Input: part model. Units: mm. Frame: model coordinates. A direction names the side the tool comes from. Give positions to 0.01 mm unless a question says otherwise; leave off trailing zeros. Order: outer loops, then holes, each group sorted by start corner. A loop starts at its lowest first (then second) coordinate and runs counter-clockwise, first axis right, second up.
```python
from build123d import *

# Parameters (mm, degrees)
SKETCH_1_W                       = 167
SKETCH_1_H                       = 155
EXTRUDE_1_DEPTH                  = 4
FILLET_1_R                       = 9
FILLET_2_R                       = 18
CUT_EXTRUDE_1_REACH              = 115.993
HOLE_WIZARD_1_D                  = 5
HOLE_WIZARD_1_CBORE_D            = 8
HOLE_WIZARD_1_CBORE_DEPTH        = 1
EXTRUDE_3_DEPTH                  = 15
CUT_EXTRUDE_2_REACH              = 146.177
SKETCH_13_W                      = 6.5
SKETCH_13_H                      = 23
SKETCH_15_W                      = 8
SKETCH_15_H                      = 3
CUT_EXTRUDE_3_DEPTH              = 2.5
FILLET_3_R                       = 0.5
PATTERN_CIRCULAR_1_COUNT         = 4
FILLET_3_OF_PATTERN_CIRCULAR_1_R = 0.5
SKETCH_18_W                      = 10
SKETCH_18_H                      = 20
EXTRUDE_4_DEPTH                  = 2
FILLET_4_R                       = 1
FILLET_4_OF_MIRROR_1_R           = 1


with BuildPart() as part:
    # ｽｹｯﾁ1 → ﾎﾞｽ - 押し出し1 (new body)
    with BuildSketch(Plane.XY):
        Rectangle(SKETCH_1_W, SKETCH_1_H)
    extrude(amount=EXTRUDE_1_DEPTH)

    # ﾌｨﾚｯﾄ1
    fillet_1_edges = [part.edges().sort_by_distance(p)[0] for p in [
        (83.5, -77.5, 2),
        (83.5, 77.5, 2),
    ]]
    fillet(fillet_1_edges, radius=FILLET_1_R)

    # ﾌｨﾚｯﾄ2
    fillet_2_edges = [part.edges().sort_by_distance(p)[0] for p in [
        (-83.5, -77.5, 2),
        (-83.5, 77.5, 2),
    ]]
    fillet(fillet_2_edges, radius=FILLET_2_R)

    # ｽｹｯﾁ2 → ｶｯﾄ - 押し出し1 (cut, up to next)
    with BuildSketch(Plane.XY.offset(4), mode=Mode.PRIVATE) as cut_extrude_1_sk1:
        with BuildLine():
            Line((58.5, 77.5), (68.5, 77.5))
            Line((68.5, 77.5), (68.5, 72.5))
            ThreePointArc((68.5, 72.5), (63.5, 67.5), (58.5, 72.5))
            Line((58.5, 72.5), (58.5, 77.5))
        make_face()
    cut_extrude_1_tool1 = extrude(cut_extrude_1_sk1.sketch, amount=-CUT_EXTRUDE_1_REACH, mode=Mode.PRIVATE) & part.part
    add(cut_extrude_1_tool1.solids().sort_by_distance((63.5, 72.966749, 4))[0], mode=Mode.SUBTRACT)

    # 穴1 (through all)
    with Locations(Plane.XY.offset(4)):
        with Locations((66, 0)):
            CounterBoreHole(HOLE_WIZARD_1_D / 2, HOLE_WIZARD_1_CBORE_D / 2, HOLE_WIZARD_1_CBORE_DEPTH)

    # ｽｹｯﾁ11 → ﾎﾞｽ - 押し出し3 (add)
    with BuildSketch(Plane.XY.offset(4)):
        with BuildLine():
            Line((36.582099448, 12), (36.582099448, -12))
            ThreePointArc((36.582099448, -12), (-38.5, 0), (36.582099448, 12))
        make_face()
        with BuildLine():
            Line((34.641016151, 11.5), (34.641016151, -11.5))
            ThreePointArc((34.641016151, -11.5), (-36.5, 0), (34.641016151, 11.5))
        make_face(mode=Mode.SUBTRACT)
    extrude(amount=EXTRUDE_3_DEPTH)

    # ｽｹｯﾁ13 → ｶｯﾄ - 押し出し2 (cut, up to next)
    with BuildSketch(Plane(origin=(36.582099448, 0, 0), x_dir=(0, 0, -1), z_dir=(1, 0, 0)), mode=Mode.PRIVATE) as cut_extrude_2_sk1:
        with Locations((-13.75, 0)):
            Rectangle(SKETCH_13_W, SKETCH_13_H)
    cut_extrude_2_tool1 = extrude(cut_extrude_2_sk1.sketch, amount=-CUT_EXTRUDE_2_REACH, mode=Mode.PRIVATE) & part.part
    add(cut_extrude_2_tool1.solids().sort_by_distance((36.582099, 0, 13.75))[0], mode=Mode.SUBTRACT)

    # ｽｹｯﾁ15 → ｶｯﾄ - 押し出し3 (cut)
    with BuildSketch(Plane(origin=(-24.72592031, 24.748737342, 1.062480514), x_dir=(0.7076465964640425, 0.7064548659887622, 0.012562517011201728), z_dir=(-0.7064548659887622, 0.7071067811865462, 0.030356586119027387))):
        with Locations((0, -14.290598152)):
            Rectangle(SKETCH_15_W, SKETCH_15_H)
    cut_extrude_3 = extrude(amount=CUT_EXTRUDE_3_DEPTH, mode=Mode.SUBTRACT)

    # ﾌｨﾚｯﾄ3
    fillet_3_edges = [part.edges().sort_by_distance(p)[0] for p in [
        (-26.293687817, 26.037155642, 16.920446126),
        (-26.331375368, 26.1282254, 13.922065571),
    ]]
    fillet(fillet_3_edges, radius=FILLET_3_R)

    # 円形ﾊﾟﾀｰﾝ1: ｶｯﾄ - 押し出し3 ×4 about axis
    pattern_circular_1_axis = Axis((0, 0, 0), (0, 0, 1))
    for i in range(1, PATTERN_CIRCULAR_1_COUNT):
        add(cut_extrude_3.rotate(pattern_circular_1_axis, i * 360 / PATTERN_CIRCULAR_1_COUNT), mode=Mode.SUBTRACT)

    # ﾌｨﾚｯﾄ3 of 円形ﾊﾟﾀｰﾝ1
    fillet_3_of_pattern_circular_1_edges = [part.edges().sort_by_distance(p)[0] for p in [
        (-26.037155642, -26.293687817, 16.920446126),
        (-26.1282254, -26.331375368, 13.922065571),
        (26.293687817, -26.037155642, 16.920446126),
        (26.331375368, -26.1282254, 13.922065571),
        (26.037155642, 26.293687817, 16.920446126),
        (26.1282254, 26.331375368, 13.922065571),
    ]]
    fillet(fillet_3_of_pattern_circular_1_edges, radius=FILLET_3_OF_PATTERN_CIRCULAR_1_R)

    # ｽｹｯﾁ18 → ﾎﾞｽ - 押し出し4 (add)
    with BuildSketch(Plane(origin=(0, 0, 0), x_dir=(-1, 0, 0), z_dir=(0, 0, -1))):
        with Locations((-82.5, 45)):
            Rectangle(SKETCH_18_W, SKETCH_18_H)
    extrude_4 = extrude(amount=EXTRUDE_4_DEPTH)

    # ﾌｨﾚｯﾄ4
    fillet_4_edges = [part.edges().sort_by_distance(p)[0] for p in [
        (77.5, 45, -2),
    ]]
    fillet(fillet_4_edges, radius=FILLET_4_R)

    # ﾐﾗｰ1: ﾎﾞｽ - 押し出し4 across plane
    add(extrude_4.mirror(Plane.ZX))

    # ﾌｨﾚｯﾄ4 of ﾐﾗｰ1
    fillet_4_of_mirror_1_edges = [part.edges().sort_by_distance(p)[0] for p in [
        (77.5, -45, -2),
    ]]
    fillet(fillet_4_of_mirror_1_edges, radius=FILLET_4_OF_MIRROR_1_R)


solid = part.part
```
1) Pull-direction query (Y, two-part tool) for faces 1 (the face through (80.794, -74.934, 2.028)), 2 (the face through (64.85, -2.22, 1.48)), 3 (the face through (-26.18, 26.06, 14.06)), 4 (the face through (35, 0, 19)); classes: pulls with the +Y half, pulls with the -Y half, needs draft (parallel to the pull), parting line crosses it, or undercut.
2) Line query: probe 1 along Z at (x, y) = (-70.5, -25); probe 2 along Y at (x, z) = (0, 8.5); probe 3 along Y at (x, z) = (66, 3.75). Output: solid intervals per line, ascending.
3) Cut plane B-B (x = 66). Return the cut outline in (y, z).
4) Reachability of faces 5 (the face through (58.5, 75, 2)), 6 (the face through (26.06, 26.18, 14.06)), 7 (the face through (83.5, -1, 2)), 8 (the face through (64, -2, 3)) from +Z, -Z, +X, -X, +Y, -Y: full face, straight path, thin tool, end or side. Return the list, or none.
5) Cut plane A-A (y = 0). Return the cut outline in (x, z).
6) First-contact query: P1, Ø2, axis at x = 35.5, z = 14, coming from the -Y side; P2, Ø5, axis at x = 18, y = 34.5, coming from the -Z side; P3, Ø3, axis at x = 84.5, y = 49.5, coming from the +Z side; P4, Ø6, axis at x = -39.5, z = 5, coming from the -Y side. Flat tips, straight axial feed; report the tip coordinate or a pass-through.
7) Cut plane D-D (y = 49). Return the cut outline in (x, z).
8) Cut plane C-C (x = 0). Return the cut outline in (y, z).
Geometry says:
1. face 1: pulls with the -Y half
1. face 2: undercut
1. face 3: undercut
1. face 4: needs draft
2. probe 1: z = 0 to 4
2. probe 2: y = -38.5 to -36.5, 36.5 to 38.5
2. probe 3: y = -77.5 to -4, 4 to 68.17
3. outline: (-77.5, 0) - (-2.5, 0) - (-2.5, 3) - (-4, 3) - (-4, 4) - (-77.5, 4) - close; (2.5, 0) - (68.17, 0) - (68.17, 4) - (4, 4) - (4, 3) - (2.5, 3) - close
4. face 5: +Z, -Z, +Y
4. face 6: none
4. face 7: +Z, +X, +Y, -Y
4. face 8: +Z
5. outline: (-83.5, 0) - (63.5, 0) - (63.5, 3) - (62, 3) - (62, 4) - (36.58, 4) - (36.58, 10.5) - (34.64, 10.5) - (34.64, 4) - (-36.5, 4) - (-36.5, 19) - (-38.5, 19) - (-38.5, 4) - (-83.5, 4) - close; (34.64, 17) - (36.58, 17) - (36.58, 19) - (34.64, 19) - close; (68.5, 0) - (83.5, 0) - (83.5, 4) - (70, 4) - (70, 3) - (68.5, 3) - close
6. P1: stops at y = -17.09
6. P2: stops at z = 0
6. P3: stops at z = 4
6. P4: stops at y = -77.5
7. outline: (-83.5, 0) - (77.5, 0) - (77.5, -1) arc R1 ccw to (78.5, -2) - (87.5, -2) - (87.5, 0) - (83.5, 0) - (83.5, 4) - (-83.5, 4) - close
8. outline: (-77.5, 0) - (77.5, 0) - (77.5, 4) - (38.5, 4) - (38.5, 19) - (36.5, 19) - (36.5, 4) - (-36.5, 4) - (-36.5, 19) - (-38.5, 19) - (-38.5, 4) - (-77.5, 4) - close
